The figure shows three views and two pictorial views of one solid part (mm, origin at its lowest corner). Answer the questions. A direction names the side the tool comes from. Coordinates: 2 decimals unless noted, no trailing zeros. Loops run counter-clockwise (first coordinate to the right, second up) from the corner with the lowest first, then second, coordinate; pieces in that order, holes last. Notation, with made-up numbers: M 29,69.25 L 76,69.25 A16 cw 76,94.25 Z; hole C -19.75,21.5 d7. An arc over 180 degrees is marked long. Return JSON: item names as keys, results as strings. Group by question number.
1. Section C-C (x = 61) is taken. Write down the section's boundary in (y, z) (3 decimals).
2. Section B-B (z = 52) is taken. Write down the section's boundary in (x, y) (3 decimals), then the cut area to 3 significant figures.
3. Given P1, Ø4, axis at x = 6.35, z = 6.35, coming from the -Y side (3 decimals); P2, Ø5, axis at x = 39, z = 17, coming from the -Y side (3 decimals); P3, Ø1.5, axis at y = 18.5, z = 35, coming from the -X side (3 decimals), each flat-ended and moving along its own axis, determine where each tip first touches the part or whether it passes through.
4. Straight lines are drawn through the part: L1, parallel to Z at x = 76, y = 46; L2, parallel to Z at x = 6, y = 46. For each, find the intervals that lie inside material, in ascending order. Write a range as from..to.
5. Section A-A (x = 42) is taken. Write down the section's boundary in (y, z) (3 decimals).
6. Which of the six approach directions +Z, -Z, +X, -X, +Y, -Y give full straight-line access (tool end or side, diameter ignored) to the marked faces 1 and 2?
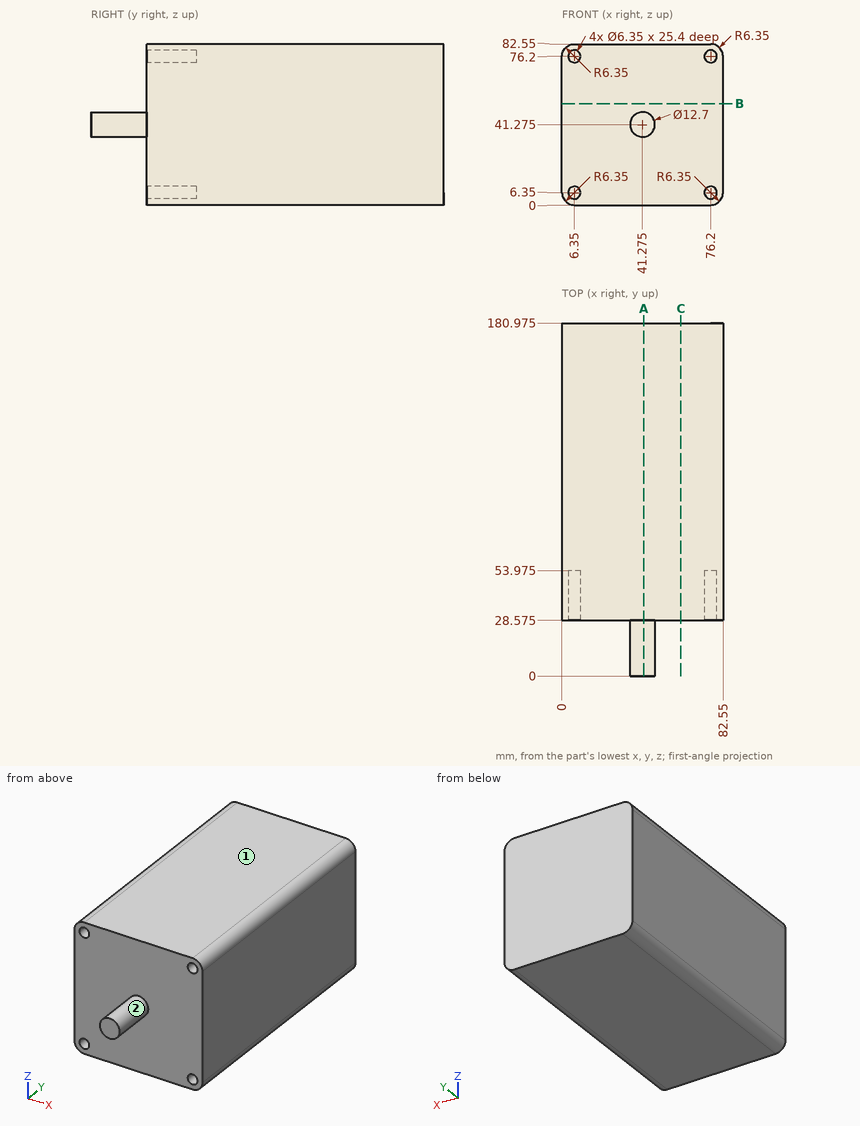
Worked out:
{
 "1": {"outline": "M 28.575,0 L 180.975,0 L 180.975,82.55 L 28.575,82.55 Z"},
 "2": {"outline": "M 0,28.575 L 82.55,28.575 L 82.55,180.975 L 0,180.975 Z", "area": "12,600 mm^2"},
 "3": {"P1": "y = 53.975", "P2": "y = 28.575", "P3": "x = 38.145"},
 "4": {"L1": "0..3.18, 9.52..73.03, 79.37..82.55", "L2": "0.01..3.19, 9.51..73.04, 79.36..82.54"},
 "5": {"outline": "M 0,34.967 L 28.575,34.967 L 28.575,0 L 180.975,0 L 180.975,82.55 L 28.575,82.55 L 28.575,47.583 L 0,47.583 Z"},
 "6": {"face 1": "+Z, +X, -X, +Y, -Y", "face 2": "-Y"}
}
